Could you check a few things on this drawing? It's one solid part, dimensions in mm from its lowest x, y, z. A direction names the side the tool comes from. Give positions to 0.01 mm unless a question says otherwise; leave off trailing zeros. Loops run counter-clockwise (first coordinate to the right, second up) from the corner with the lowest first, then second, coordinate; pieces in that order, holes last.
1. Imagine slicing it at C-C (z = 2.2). List the corners of the cut face in (x, y) for me (1 decimal).
2. I need wall thicknesses on line 1 along X through (y, z) = (6.5, 1.7) (1 decimal); line 2 along X through (y, z) = (7.75, 2.3) (1 decimal); line 3 along Y through (x, z) = (12, 1.6) (1 decimal). Which ranges of each line are inside material? Lowest first, please.
3. Imagine slicing it at A-A (x = 11). List the corners of the cut face in (y, z) for me.
4. For the marked faces 4, 5 and 6, which set-ups out of +Z, -Z, +X, -X, +Y, -Y let a thin tool reach every point of the face, with its end or its side?
5. Imagine slicing it at B-B (y = 6.5). List the corners of the cut face in (x, z) for me.
6. Thinking about a two-plate mould opening in X: for the marked faces 1, 2 and 3, which applies, +X half, -X half, draft (parallel to the pull), parting line (faces both ways), or undercut?
7. Imagine slicing it at D-D (y = 10). List the corners of the cut face in (x, z) for me.
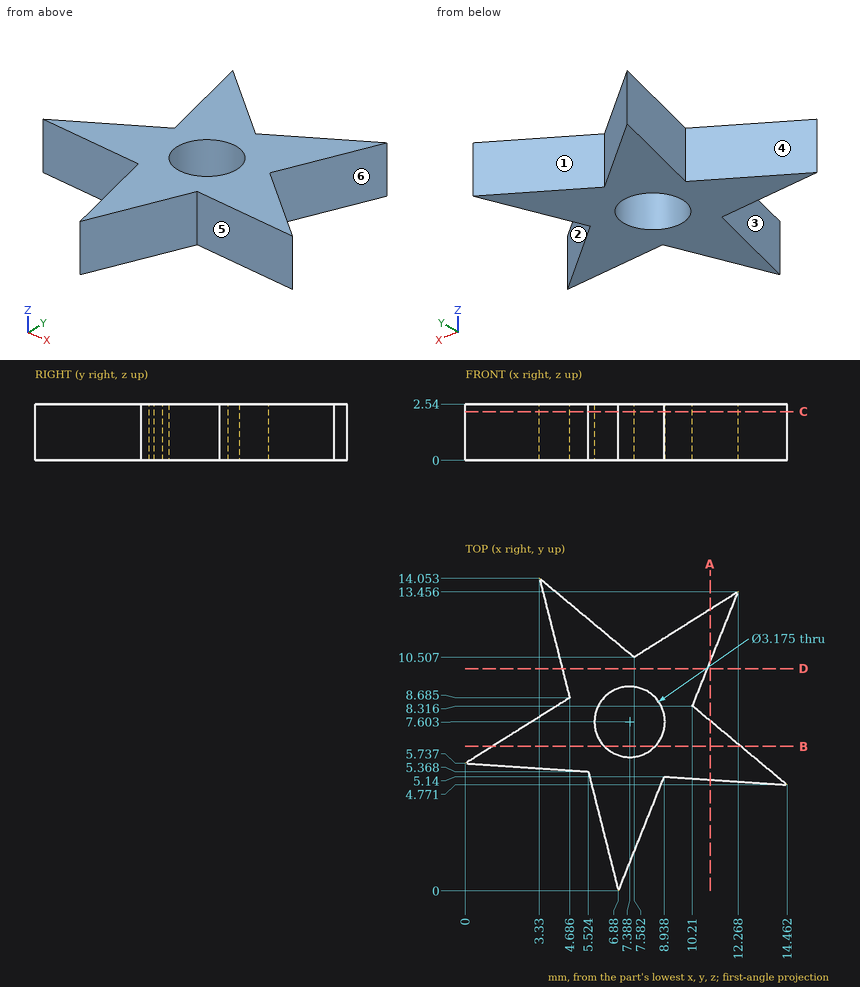
Derived:
1. outline: (0, 5.7) - (5.5, 5.4) - (6.9, 0) - (8.9, 5.1) - (14.5, 4.8) - (10.2, 8.3) - (12.3, 13.5) - (7.6, 10.5) - (3.3, 14.1) - (4.7, 8.7) - close; hole circle Ø3.2 at (7.4, 7.6)
2. line 1: x = 1.2 to 6.2, 8.5 to 12.4
2. line 2: x = 3.2 to 5.8, 9 to 10.9
2. line 3: y = 4.9 to 6.8, 12.8 to 13.3
3. outline: (5, 0) - (7.66, 0) - (7.66, 2.54) - (5, 2.54) - close; (10.29, 0) - (12.66, 0) - (12.66, 2.54) - (10.29, 2.54) - close
4. face 4: +Z, -Z, -X
4. face 5: +Z, -Z, -Y
4. face 6: +Z, -Z, +X
5. outline: (1.21, 0) - (6.25, 0) - (6.25, 2.54) - (1.21, 2.54) - close; (8.53, 0) - (12.39, 0) - (12.39, 2.54) - (8.53, 2.54) - close
6. face 1: undercut
6. face 2: +X half
6. face 3: -X half
7. outline: (4.35, 0) - (10.88, 0) - (10.88, 2.54) - (4.35, 2.54) - close
